from build123d import *

# Parameters (mm, degrees)
SKETCH4_R           = 34
SKETCH4_R_2         = 24
SKETCH4_R_3         = 2
BOSS_EXTRUDE1_DEPTH = 9


with BuildPart() as part:
    # Sketch1 → Revolve1 (revolve)
    with BuildSketch(Plane.XY):
        Polygon((-12, 8), (-12, -8), (-16, -8), (-16, -24), (-20, -24), (-20, -38), (-24, -38), (-24, 38), (-20, 38), (-20, 24), (-16, 24), (-16, 8), align=None)
    revolve(axis=Axis((0, 75.096781517, 0), (0, -1, 0)))

    # Sketch4 → Boss-Extrude1 (add)
    with BuildSketch(Plane(origin=(0, 38, 0), x_dir=(1, 0, 0), z_dir=(0, 1, 0))):
        Circle(SKETCH4_R)
        Circle(SKETCH4_R_2, mode=Mode.SUBTRACT)
        with Locations((0, 29)):
            Circle(SKETCH4_R_3, mode=Mode.SUBTRACT)
        with Locations((20.506096654, 20.506096654)):
            Circle(SKETCH4_R_3, mode=Mode.SUBTRACT)
        with Locations((29, 0)):
            Circle(SKETCH4_R_3, mode=Mode.SUBTRACT)
        with Locations((20.506096654, -20.506096654)):
            Circle(SKETCH4_R_3, mode=Mode.SUBTRACT)
        with Locations((0, -29)):
            Circle(SKETCH4_R_3, mode=Mode.SUBTRACT)
        with Locations((-20.506096654, -20.506096654)):
            Circle(SKETCH4_R_3, mode=Mode.SUBTRACT)
        with Locations((-29, 0)):
            Circle(SKETCH4_R_3, mode=Mode.SUBTRACT)
        with Locations((-20.506096654, 20.506096654)):
            Circle(SKETCH4_R_3, mode=Mode.SUBTRACT)
    boss_extrude1 = extrude(amount=-BOSS_EXTRUDE1_DEPTH)

    # Mirror1: Boss-Extrude1 across plane
    add(boss_extrude1.mirror(Plane.ZX))


solid = part.part
Check sheet for the modelled part. Datum: model origin and axes. Units: mm. A direction names the side the tool comes from. Coordinates: 2 decimals unless noted, no trailing zeros. Write each loop counter-clockwise with the first axis right and the second up, starting at its lowest first coordinate (ties: lowest second). Pieces come first, ordered by that corner, then holes. Notation, with made-up numbers: M -36.75,29 L -1.75,29 A19 cw -1.75,57 Z; hole C 15.25,66 d10. An arc over 180 degrees is marked long. Answer as CSV lines item,"result".
Q1. Cross-section at C-C (y = 4.5). Record the boundary of the cut face in (x, z).
Check result:
outline,"C 0,0 d48; hole C 0,0 d24"
Q2. Go/stop test with flat-tipped pins: pin 1 (12 mm diameter, centred on x = 5.5, z = -4.5, fed in from +Y); pin 2 (5 mm diameter, centred on x = 0, z = -29, fed in from -Y); pin 3 (10 mm diameter, centred on x = -2, y = 22, fed in from -Z); pin 4 (1 mm diameter, centred on x = 22, y = -15.5, fed in from +Z). Record where each tip stops, or that it passes through.
Check result:
pin 1,"y = 8"
pin 2,"y = -38"
pin 3,"z = -24"
pin 4,"z = 10.67"
Q3. Mould release check, pull along Z, two halves, no side actions. Record for faces 5 (the face through (18.28, 33.56, -28.67)), 6 (the face through (20.25, -33.56, -22.49)), 7 (the face through (-8, 29, -23)): released by +Z, released by -Z, zero draft, split by the parting line, or undercut.
Check result:
face 5,"split by the parting line"
face 6,"undercut"
face 7,"zero draft"
Q4. Cross-section at B-B (x = -29). Record the boundary of the cut face in (y, z), then the cut area to 3 significant figures.
Check result:
outline,"M -38,-17.75 L -29,-17.75 L -29,-2 L -38,-2 Z; M -38,2 L -29,2 L -29,17.75 L -38,17.75 Z; M 29,-17.75 L 38,-17.75 L 38,-2 L 29,-2 Z; M 29,2 L 38,2 L 38,17.75 L 29,17.75 Z"
area,"567 mm^2"
Q5. Cross-section at D-D (z = 0). Count the separate pieces of the cut face and the enclosed holes in it, then the cut area to 3 significant figures.
Check result:
separate pieces,"6"
enclosed holes,"0"
area,"1,340 mm^2"
Q6. Material ranges on probe 1 along Z at (x, y) = (0, 31.75); probe 2 along Y at (x, z) = (-30, -12), recorded low to high. Write a range as from..to.
Check result:
probe 1,"-34..-31, -27..-20, 20..27, 31..34"
probe 2,"-38..-29, 29..38"
Q7. Set-up check for faces 1 (the face through (-8, -29, -23)), 2 (the face through (4.336, 30.902, 19.524)), 3 (the face through (3.47, -16.11, 15.62)), 4 (the face through (11.99, -0.11, -0.53)): record each of +Z, -Z, +X, -X, +Y, -Y from which the full face is reachable in a straight line by a thin tool's end or side.
Check result:
face 1,"none"
face 2,"+Y"
face 3,"-Y"
face 4,"+Y, -Y"
Q8. Cross-section at A-A (z = -26). Record the boundary of the cut face in (x, y).
Check result:
outline,"M -21.91,-38 L 21.91,-38 L 21.91,-29 L -21.91,-29 Z; M -21.91,29 L 21.91,29 L 21.91,38 L -21.91,38 Z"
